Job drawing, mm, ordinate dimensions from the low corner. One solid piece. Give positions to 0.01 mm unless a question says otherwise; leave off trailing zeros. Write each loop counter-clockwise with the first axis right and the second up, starting at its lowest first coordinate (ties: lowest second). Pieces come first, ordered by that corner, then holes. Notation, with made-up numbers: (23.5, -37.5) - (60.5, -37.5) arc R11 ccw to (60.5, -16.5) - close; hole circle Ø7 at (-1, -27.5). An arc over 180 degrees is marked (long way). Answer as a JSON object with one key per item and string values.
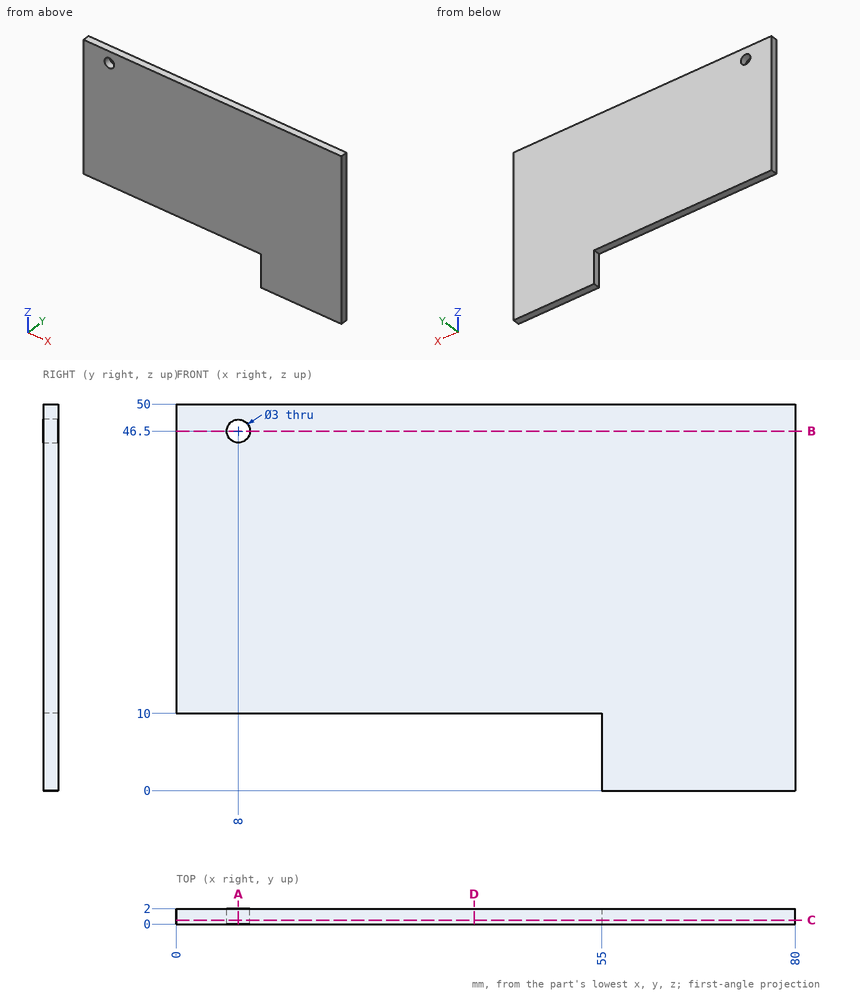
Item 1: Cut at C-C (y = 0.5). Give the cut face in (x, z).
Entries:
{"outline": "(0, 10) - (55, 10) - (55, 0) - (80, 0) - (80, 50) - (0, 50) - close; hole circle Ø3 at (8, 46.5)"}
Item 2: Cut at D-D (x = 38.5). Give the cut face in (y, z).
Entries:
{"outline": "(0, 10) - (2, 10) - (2, 50) - (0, 50) - close"}
Item 3: Probe line 1 (X direction, y = 0.9, z = 46.5); line 2 (X direction, y = 1.3, z = 7.5); line 3 (Z direction, x = 40.5, y = 1.6). List the from-to ranges inside material, lowest first. Write a range as from..to.
Entries:
{"line 1": "0..6.5, 9.5..80", "line 2": "55..80", "line 3": "10..50"}
Item 4: Cut at B-B (z = 46.5). Give the cut face in (x, y), and give its area (3 significant figures).
Entries:
{"outline": "(0, 0) - (6.5, 0) - (6.5, 2) - (0, 2) - close; (9.5, 0) - (80, 0) - (80, 2) - (9.5, 2) - close", "area": "154 mm2"}
Item 5: Cut at A-A (x = 8). Give the cut face in (y, z).
Entries:
{"outline": "(0, 10) - (2, 10) - (2, 45) - (0, 45) - close; (0, 48) - (2, 48) - (2, 50) - (0, 50) - close"}
